Can you work these out from the model? Positions are in its coordinate system, mm. A direction names the side the tool comes from. Coordinates: 2 decimals unless noted, no trailing zeros. Loops run counter-clockwise (first coordinate to the right, second up) from the corner with the lowest first, then second, coordinate; pieces in that order, holes last.
```python
from build123d import *

# Parameters (mm, degrees)
F0_W     = 152.4
F0_H     = 76.2
F1_DEPTH = 76.2
F3_DEPTH = 76.2
F5_DEPTH = 152.4


with BuildPart() as f1:
    # F0 (on Front) → F1 (new body)
    with BuildSketch(Plane.XZ):
        with Locations((26.298277, -38.1)):
            Rectangle(F0_W, F0_H)
    extrude(amount=F1_DEPTH)

    # F2 (on face) → F3 (cut)
    with BuildSketch(Plane.XZ.offset(76.2)):
        Polygon((0, 0), (-24.501723, 0), (-24.501723, -12.7), (-37.201723, -12.7), (-37.201723, -25.4), (13.598277, -25.4), (13.598277, -12.7), (0.898277, -12.7), align=None)
        Polygon((32.648277, -12.7), (102.498277, -12.7), (102.498277, 0), (26.298277, 0), align=None)
    extrude(amount=-F3_DEPTH, mode=Mode.SUBTRACT)

    # F4 (on face) → F5 (cut, through all)
    with BuildSketch(Plane.YZ.offset(102.498277)):
        Polygon((-50.8, -76.2), (-25.4, -76.2), (-12.7, -63.5), (-63.5, -63.5), align=None)
    extrude(amount=-F5_DEPTH, mode=Mode.SUBTRACT)


solid = f1.part
```
Item 1: Suppose I cut it at C-C, the plane x = 6. Please give me the cut outline in (y, z), plus the area to 3 significant figures.
Results are:
outline: (-76.2, -76.2) - (-50.8, -76.2) - (-63.5, -63.5) - (-12.7, -63.5) - (-25.4, -76.2) - (0, -76.2) - (0, -25.4) - (-76.2, -25.4) - close; (-76.2, -12.7) - (0, -12.7) - (0, 0) - (-76.2, 0) - close
area: 4,350 mm2
Item 2: Suppose I cut it at D-D, the plane x = 86. Please give me the cut outline in (y, z), plus the area to 3 significant figures.
Results are:
outline: (-76.2, -76.2) - (-50.8, -76.2) - (-63.5, -63.5) - (-12.7, -63.5) - (-25.4, -76.2) - (0, -76.2) - (0, -12.7) - (-76.2, -12.7) - close
area: 4,350 mm2
Item 3: I'm going to push flat-ended pins straight in: P1, Ø15, axis at x = -8.5, y = -33, coming from the +Z side; P2, Ø4, axis at y = -42.5, z = -8, coming from the +X side; P3, Ø15, axis at x = 34, y = -40.5, coming from the -Z side. Where does each tip first touch, or does it pass through?
Results are:
P1: stops at z = -25.4
P2: stops at x = 31.3
P3: stops at z = -63.5
Item 4: Suppose I cut it at B-B, the plane z = -22. Please give me the cut outline in (x, y).
Results are:
outline: (-49.9, -76.2) - (-37.2, -76.2) - (-37.2, 0) - (-49.9, 0) - close; (13.6, -76.2) - (102.5, -76.2) - (102.5, 0) - (13.6, 0) - close
Item 5: Suppose I cut it at A-A, the plane y = -19.5. Please give me the cut outline in (x, z), plus the area to 3 significant figures.
Results are:
outline: (-49.9, -76.2) - (102.5, -76.2) - (102.5, -70.3) - (-49.9, -70.3) - close; (-49.9, -63.5) - (102.5, -63.5) - (102.5, -12.7) - (32.65, -12.7) - (26.3, 0) - (0, 0) - (0.9, -12.7) - (13.6, -12.7) - (13.6, -25.4) - (-37.2, -25.4) - (-37.2, -12.7) - (-24.5, -12.7) - (-24.5, 0) - (-49.9, 0) - close
area: 8,690 mm2
Item 6: I need wall thicknesses on line 1 along X through (y, z) = (-58, -19.5); line 2 along Z through (x, y) = (-28, -72); line 3 along Z through (x, y) = (13.5, -35). Which ranges of each line are inside material? Lowest first, please.
Results are:
line 1: x = -49.9 to -37.2, 13.6 to 102.5
line 2: z = -76.2 to -25.4, -12.7 to 0
line 3: z = -63.5 to -25.4, -12.7 to 0
Item 7: On a 3-axis mill with a long thin cutter (end or side, diameter ignored), from which of +Z, -Z, +X, -X, +Y, -Y can I reach the whole of each face in a straight line? I mean faces 4 (the face through (67, -39, -12.7)), 5 (the face through (27, -38, -63.5)), 6 (the face through (7, -39, -12.7)), 7 (the face through (25, -13, -76.2)). Say none if no direction works.
Results are:
face 4: +Z, +X, +Y, -Y
face 5: +X, -X
face 6: +Y, -Y
face 7: -Z, +X, -X, +Y, -Y
Item 8: We'd pull the mould along Y, two halves only. Please class faces 1 (the face through (25, 0, -46)), 2 (the face through (-37.202, -39, -19)), 3 (the face through (27.4, -19.1, -69.9)): +Y half, -Y half, draft (parallel to the pull), parting line (faces both ways), or undercut.
Results are:
face 1: +Y half
face 2: draft
face 3: undercut
